For this review, take the finished solid that the model builds, in its own axes (mm). Coordinates: 2 decimals unless noted, no trailing zeros. Order: outer loops, then holes, each group sorted by start corner. A loop starts at its lowest first (then second) coordinate and runs counter-clockwise, first axis right, second up. Notation, with made-up numbers: (38.25, 7.25) -> (54.25, 7.25) arc R14 cw to (54.25, 29.25) -> close; hole circle Ø11 at (73.25, 35.25). An arc over 180 degrees is marked (long way). Return JSON: item names as keys, results as strings. Group by question number.
Item 1: For line 1 along Y through (x, z) = (10, 2); line 2 along Y through (x, z) = (10, 6); line 3 along Y through (x, z) = (10, 6.25), list the stretches that pass through material, from the lowest coordinate up.
Item 2: Take a section at C-C (z = 4.5). Count the separate pieces of the cut face and the enclosed holes in it, then the cut area to 3 significant figures.
Item 3: Insertion check: pin 1 (5 mm diameter, centred on x = 15.5, z = 4.5, fed in from +Y); pin 2 (1.5 mm diameter, centred on x = 16.5, z = 1, fed in from +Y). Each pin has a flat end and moves straight along its axis. Give the tip position at first contact, or say it passes through.
Item 4: Take a section at A-A (x = 10). Write out the cut boundary in (y, z), then the cut area to 3 significant figures.
Item 5: Take a section at B-B (z = 2.25). Write out the cut boundary in (x, y).
Autodesk Fusion 360 part; units mm, degrees
sketch "Esquisse1" plane through (0, 0, 0) normal (0, 0, 1) x (1, 0, 0)
  line L0 (7, 0) -> (13, 0)
  line L1 (20, 7) -> (20, 21)
  line L2 (13, 28) -> (7, 28)
  line L3 (0, 21) -> (0, 7)
  line L4 (10, 28) -> (10, 0) construction
  circle A0 centre (10, 23.45) radius 2.1
  circle A1 centre (10, 4.55) radius 2.1
  line L5 (-6, 20) -> (25, 20) construction
  line L6 (25, 20) -> (25, 8) construction
  line L7 (25, 8) -> (-6, 8) construction
  line L8 (-6, 8) -> (-6, 20) construction
  line L9 (13, 0) -> (20, 7)
  line L10 (7, 0) -> (0, 7)
  line L11 (20, 21) -> (13, 28)
  line L12 (7, 28) -> (0, 21)
  point P0 (20, 0)
  point P1 (20, 28)
  point P2 (0, 28)
  dimension "d1" = 20
  dimension "d2" = 28
  dimension "d3" = 4.2
  dimension "d4" = 4.2
  dimension "d5" = 18.9
  dimension "d6" = 4.55
  dimension "d7" = 12
  dimension "d8" = 8
  dimension "d9" = 7
  dimension "d10" = 7
  dimension "d11" = 7
  dimension "d12" = 7
  dimension "d13" = 7
  dimension "d14" = 7
  dimension "d15" = 7
  dimension "d16" = 7
extrude "Extrusion1" add sketch "Esquisse1" along normal blind 9
sketch "Esquisse2" plane through (20, 0, 0) normal (1, 0, 0) x (0, 1, 0)
  line L0 (7, 0) -> (21, 0)
  line L1 (21, 0) -> (21, 9)
  line L2 (21, 9) -> (7, 9)
  line L3 (7, 9) -> (7, 0)
  circle A0 centre (14, 10) radius 6
  dimension "d19" = 12
  dimension "d20" = 10
  dimension "d21" = 7
extrude "Extrusion2" cut sketch "Esquisse2" against normal blind 20 contours L2 A0 | L2 A0
chamfer "Chanfrein1" distance 1.5 angle 45 8 edges at (16.5, 3.5, 0) (20, 14, 0) (16.5, 24.5, 0) (10, 28, 0) (3.5, 24.5, 0) (0, 14, 0) (3.5, 3.5, 0) (10, 0, 0)
fillet "Congé1" radius 0.5 22 edges at (10, 8.0839, 9) (10, 19.9161, 9) (0, 21, 5.25) (0, 7, 5.25) (0, 7.542, 9) (7, 0, 5.25) (13, 0, 5.25) (20, 7, 5.25) (20, 7.542, 9) (20, 14, 4) (0, 14, 4) (3.5, 24.5, 9) (10, 28, 9) (16.5, 24.5, 9) (20, 20.458, 9) (0, 20.458, 9) (20, 21, 5.25) (13, 28, 5.25) (7, 28, 5.25) (16.5, 3.5, 9) (10, 0, 9) (3.5, 3.5, 9)
fillet "Congé2" radius 0.5 8 edges at (0.769, 7.3185, 0.731) (7.3185, 0.769, 0.731) (12.6815, 0.769, 0.731) (0.769, 20.6815, 0.731) (7.3185, 27.231, 0.731) (12.6815, 27.231, 0.731) (19.231, 20.6815, 0.731) (19.231, 7.3185, 0.731)
equation "d5 = 14.7 mm + 4.2 mm"
equation "d6 = ( ( 28 - 18.9 ) / 2 ) * 1 mm"
equation "d10 = d9"
equation "d12 = d11"
equation "d14 = d13"
equation "d16 = d15"
Findings below:
{
 "1": {"line 1": "y = 0 to 2.45, 6.65 to 21.35, 25.55 to 28", "line 2": "y = 0 to 2.45, 6.65 to 9.53, 18.47 to 21.35, 25.55 to 28", "line 3": "y = 0 to 2.45, 6.65 to 9.32, 18.68 to 21.35, 25.55 to 28"},
 "2": {"separate pieces": "2", "enclosed holes": "2", "area": "338 mm2"},
 "3": {"pin 1": "stops at y = 27.96", "pin 2": "stops at y = 25.06"},
 "4": {"outline": "(0, 1.5) -> (1.5, 0) -> (2.45, 0) -> (2.45, 9) -> (0.5, 9) arc R0.5 ccw to (0, 8.5) -> close; (6.65, 0) -> (21.35, 0) -> (21.35, 9) -> (20.32, 9) arc R0.5 ccw to (19.84, 8.62) arc R6 cw to (8.16, 8.62) arc R0.5 ccw to (7.68, 9) -> (6.65, 9) -> close; (25.55, 0) -> (26.5, 0) -> (28, 1.5) -> (28, 8.5) arc R0.5 ccw to (27.5, 9) -> (25.55, 9) -> close", "area": "129 mm2"},
 "5": {"outline": "(0, 7.21) arc R0.5 ccw to (0.15, 6.85) -> (6.85, 0.15) arc R0.5 ccw to (7.21, 0) -> (12.79, 0) arc R0.5 ccw to (13.15, 0.15) -> (19.85, 6.85) arc R0.5 ccw to (20, 7.21) -> (20, 20.79) arc R0.5 ccw to (19.85, 21.15) -> (13.15, 27.85) arc R0.5 ccw to (12.79, 28) -> (7.21, 28) arc R0.5 ccw to (6.85, 27.85) -> (0.15, 21.15) arc R0.5 ccw to (0, 20.79) -> close; hole circle Ø4.2 at (10, 4.55); hole circle Ø4.2 at (10, 23.45)"}
}
